Part print with two shaded views. Sizes in mm from the minimum x, y, z corner. A direction names the side the tool comes from. Round coordinates to 2 decimals unless told otherwise and drop trailing zeros. Loops run counter-clockwise (first coordinate to the right, second up) from the corner with the lowest first, then second, coordinate; pieces in that order, holes last. Notation, with made-up numbers: (67, -18.75) -> (119, -18.75) arc R27 cw to (119, 17.25) -> close; hole circle Ø10 at (79, 22.25). An arc over 180 degrees is marked (long way). Answer as a JSON object with one key per item and string values. Group by question number.
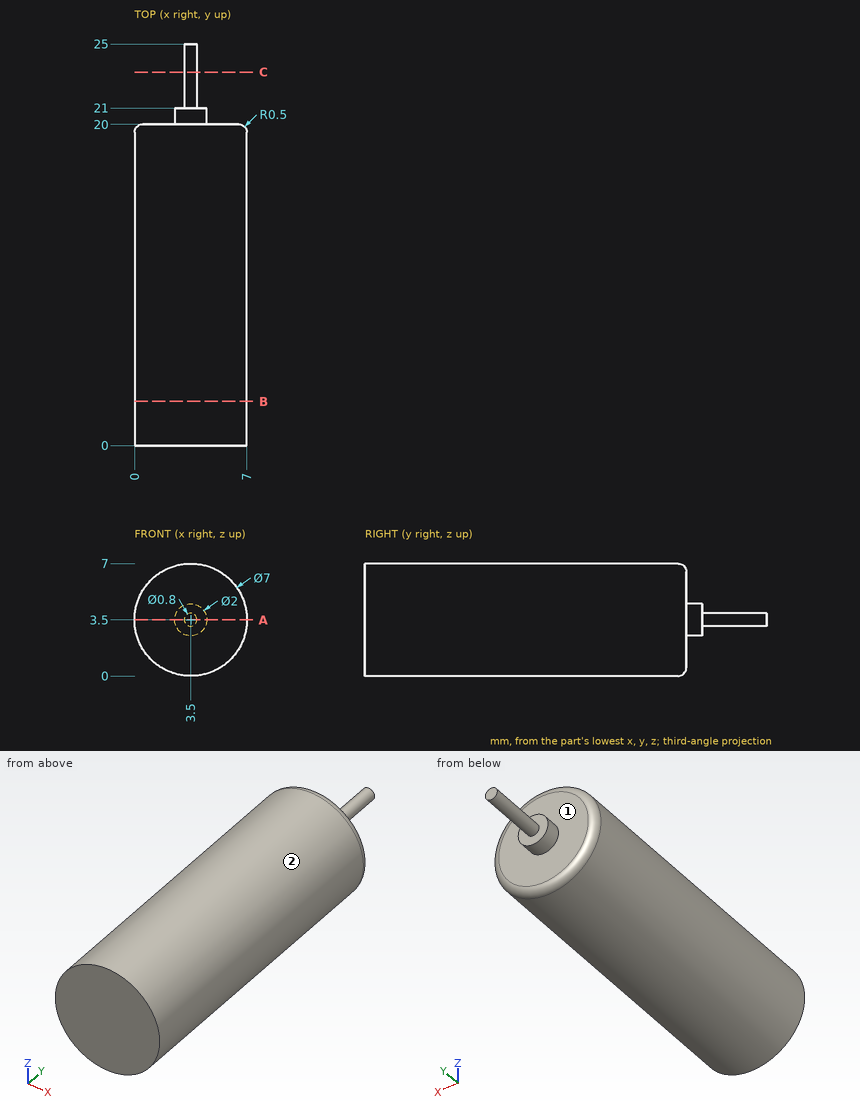
Item 1: Band-saw the part on B-B, the plane y = 2.75. List the corners of the cut face in (x, z), plus the area to 3 significant figures.
Item 2: Band-saw the part on C-C, the plane y = 23.25. List the corners of the cut face in (x, z), plus the area to 3 significant figures.
Item 3: Drop a flat-ended pin along its axis: pin 1 Ø1 at (x, z) = (4, 3.5) entering from +Y. Give the stop position or say it passes through.
Item 4: Band-saw the part on A-A, the plane z = 3.5. List the corners of the cut face in (x, y).
Item 5: Which spindle directions (+Z, -Z, +X, -X, +Y, -Y) get a long thin tool onto all of the face, cutting with end or side? Do the marked faces 1 and 2. Say none if no direction does.
Item 6: Drill centre lines: line 1 (Y direction, x = 1, z = 1.75); line 2 (Y direction, x = 6.5, z = 4.75); line 3 (Z direction, x = 3.75, y = 3.75). Where is each one in solid material? Low to high.
Entries:
{
 "1": {"outline": "circle Ø7 at (3.5, 3.5)", "area": "38.5 mm²"},
 "2": {"outline": "circle Ø0.8 at (3.5, 3.5)", "area": "0.503 mm²"},
 "3": {"pin 1": "y = 25"},
 "4": {"outline": "(0, 0) -> (7, 0) -> (7, 19.5) arc R0.5 ccw to (6.5, 20) -> (4.5, 20) -> (4.5, 21) -> (3.9, 21) -> (3.9, 25) -> (3.1, 25) -> (3.1, 21) -> (2.5, 21) -> (2.5, 20) -> (0.5, 20) arc R0.5 ccw to (0, 19.5) -> close"},
 "5": {"face 1": "+Y", "face 2": "+Y, -Y"},
 "6": {"line 1": "0 to 20", "line 2": "0 to 19.93", "line 3": "0.01 to 6.99"}
}
